Geometry: see drawing. Coordinates: mm, zero at the bounding-box minimum. Coordinates: 2 decimals unless noted, no trailing zeros. Write each loop counter-clockwise with the first axis right and the second up, starting at its lowest first coordinate (ties: lowest second). Pieces come first, ordered by that corner, then holes.
1) Section query A-A (z = 21). Output: boundary loops of the cut face in (x, y), then the cut area to 4 significant figures.
2) Line query: L1, parallel to X at y = 1.5, z = 62.5; L2, parallel to Z at x = 193, y = 4.3. Output: solid intervals per line, ascending.
3) Section query B-B (x = 103.5). Output: boundary loops of the cut face in (y, z), then the cut area to 3 significant figures.
4) Pin query (flat end, axial travel): pin 1 Ø1 at (x, y) = (192, 1.5) entering from -Z; pin 2 Ø2.5 at (y, z) = (3.5, 66.5) entering from -X; pin 3 Ø1.5 at (x, y) = (211.5, 2) entering from +Z. Return the tip coordinate at first contact, or that it passes through.
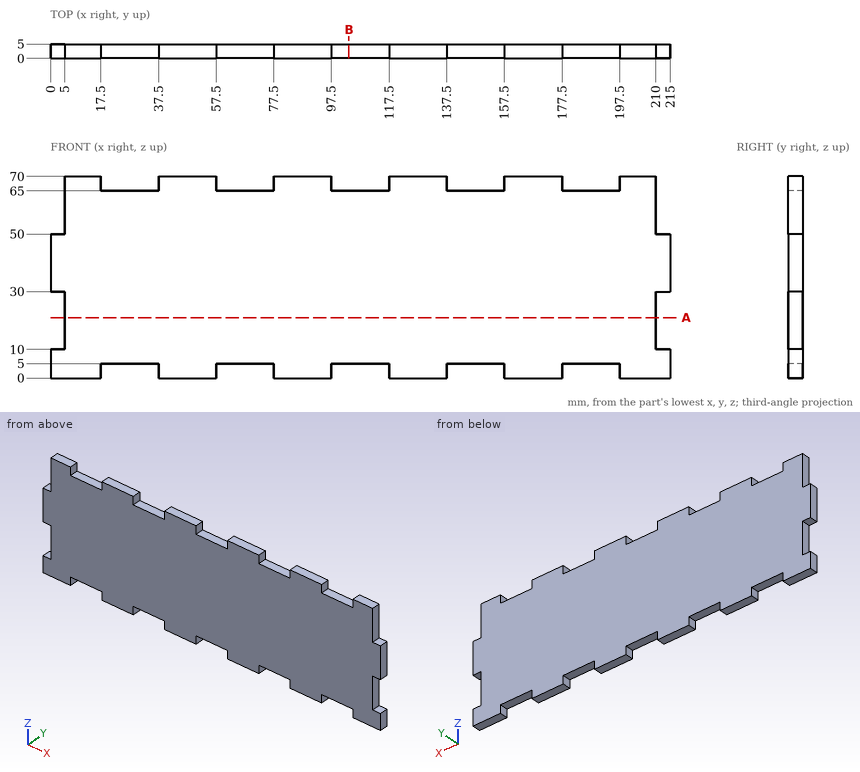
Answer:
1. outline: (5, 0) - (210, 0) - (210, 5) - (5, 5) - close
1. area: 1,025 mm2
2. L1: x = 5 to 210
2. L2: z = 5 to 65
3. outline: (0, 5) - (5, 5) - (5, 65) - (0, 65) - close
3. area: 300 mm2
4. pin 1: stops at z = 5
4. pin 2: stops at x = 5
4. pin 3: stops at z = 50
